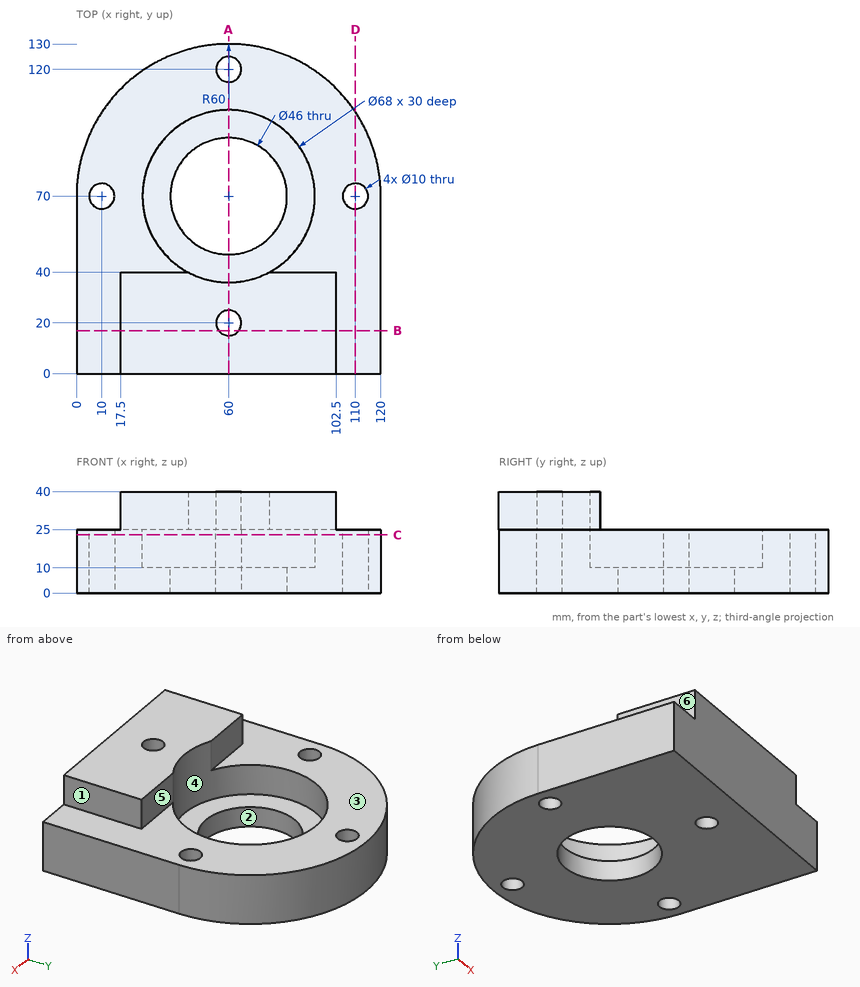
For this review, use the dimensioned drawing (mm, ordinates from the lowest corner) and the shaded views. A direction names the side the tool comes from. Round coordinates to 2 decimals unless told otherwise and drop trailing zeros. Loops run counter-clockwise (first coordinate to the right, second up) from the corner with the lowest first, then second, coordinate; pieces in that order, holes last. Notation, with made-up numbers: M 17,57.5 L 28,57.5 A37 ccw 28,96.5 Z; hole C 44,-12.75 d1. An arc over 180 degrees is marked long. Answer as a JSON object with one key per item and string values.
(1) Clearance check with flat-ended pins moving along their axes: P1, Ø6, axis at x = 60, y = 20, coming from the -Z side; P2, Ø4.5, axis at x = 31, z = 34.5, coming from the +Y side; P3, Ø1.5, axis at y = 88, z = 21, coming from the +X side; P4, Ø7.5, axis at y = 24.5, z = 29.5, coming from the -X side. State where each tip first meets the part, or that it passes through.
Resolved:
{"P1": "through", "P2": "y = 40", "P3": "x = 117.47", "P4": "x = 17.5"}
(2) Tool access review of the marked faces 4, 5 and 6: name each direction out of +Z, -Z, +X, -X, +Y, -Y from which nothing blocks a thin tool from reaching the whole face with its end or side.
Resolved:
{"face 4": "+Z", "face 5": "+Z, +X, -X, +Y", "face 6": "+Z, -X, +Y, -Y"}
(3) Take a section at A-A on x = 60. Give the boundary of the cut face in (y, z).
Resolved:
{"outline": "M 0,0 L 15,0 L 15,40 L 0,40 Z; M 25,0 L 47,0 L 47,10 L 36,10 L 36,40 L 25,40 Z; M 93,0 L 115,0 L 115,25 L 104,25 L 104,10 L 93,10 Z; M 125,0 L 130,0 L 130,25 L 125,25 Z"}
(4) Draft analysis for pull direction X (two halves, no side actions). For the marked faces 1, 2 and 3, state which applies: released by +X, released by -X, zero draft, split by the parting line, or undercut.
Resolved:
{"face 1": "released by +X", "face 2": "undercut", "face 3": "zero draft"}
(5) To check wall thickness, follow line 1 along Y through (x, z) = (60, 19.5); line 2 along Y through (x, z) = (60, 9); line 3 along X through (y, z) = (67.5, 4). State the ranges of each line that lie inside material, in increasing order.
Resolved:
{"line 1": "0 to 15, 25 to 36, 104 to 115, 125 to 130", "line 2": "0 to 15, 25 to 47, 93 to 115, 125 to 130", "line 3": "0 to 5.67, 14.33 to 37.14, 82.86 to 105.67, 114.33 to 120"}
(6) Take a section at B-B on y = 17. Give the boundary of the cut face in (x, z).
Resolved:
{"outline": "M 0,0 L 56,0 L 56,40 L 17.5,40 L 17.5,25 L 0,25 Z; M 64,0 L 120,0 L 120,25 L 102.5,25 L 102.5,40 L 64,40 Z"}
(7) Take a section at D-D on x = 110. Give the boundary of the cut face in (y, z), and give its area (3 significant figures).
Resolved:
{"outline": "M 0,0 L 65,0 L 65,25 L 0,25 Z; M 75,0 L 103.17,0 L 103.17,25 L 75,25 Z", "area": "2,330 mm²"}
(8) Take a section at C-C on z = 23. Give the boundary of the cut face in (x, y), and give its area (3 significant figures).
Resolved:
{"outline": "M 0,0 L 120,0 L 120,70 A60 ccw 0,70 Z; hole C 10,70 d10; hole C 60,70 d68; hole C 60,20 d10; hole C 60,120 d10; hole C 110,70 d10", "area": "10,100 mm²"}
